Verification items for the finished model (mm, model axes). A direction names the side the tool comes from. Round coordinates to 2 decimals unless told otherwise and drop trailing zeros. Order: outer loops, then holes, each group sorted by start corner. A loop starts at its lowest first (then second) coordinate and runs counter-clockwise, first axis right, second up. Notation, with made-up numbers: M 17.5,43.5 L 35.5,43.5 A9 ccw 35.5,59.5 Z; hole C -2.5,2 d1. An arc over 180 degrees is marked long. Write item = value, one per line. Start each with the question number.
from build123d import *

# Parameters (mm, degrees)
F0_W      = 12.7
F0_H      = 12.7
F1_DEPTH  = 50.8
F3_DEPTH  = 25.4
F5_DEPTH  = 25.4
F7_DEPTH  = 12.7
F9_DEPTH  = 25.4
F12_DEPTH = 25.4
F13_W     = 40.64
F13_H     = 7.62
F15_W     = 7.62
F15_H     = 40.64
F11_W     = 7.62
F11_H     = 40.64
F14_W     = 40.64
F14_H     = 7.62
F16_DEPTH = 43.18


# Not quite as in the source:
# - a feature names something its author has since deleted; it is built from what else it names


with BuildPart() as f1:
    # F0 (on Top) → F1 (new body)
    with BuildSketch(Plane.XY):
        Polygon((0, 12.7), (0, 0), (31.75, 0), (38.0062268819, 0), (50.8, 0), (50.8, 12.7), (38.1, 12.7), (31.75, 12.7), align=None)
        Polygon((0, -5.08), (0, 0), (-12.7, 0), (-12.7, -5.08), (-12.7, -13.97), (-12.7, -16.51), (-12.7, -25.4), (-12.7, -31.75), (-12.7, -38.1), (-12.7, -50.8), (0, -50.8), (0, -38.0530845557), (0, -31.75), (0, -25.4), (0, -16.51), (0, -13.97), align=None)
        Polygon((-12.7, 12.7), (0, 12.7), (0, 17.78), (0, 26.67), (0, 29.21), (0, 38.1), (0, 44.45), (0, 50.8), (0, 63.5), (-12.7, 63.5), (-12.7, 50.8), (-12.7, 44.45), (-12.7, 38.1), (-12.7, 26.67), (-12.7, 17.78), align=None)
        Polygon((-44.45, 0), (-12.7, 0), (-12.7, 12.7), (-44.45, 12.7), (-50.8, 12.7), (-63.5, 12.7), (-63.5, 0), (-50.8, 0), align=None)
        with Locations((-6.35, 6.35)):
            Rectangle(F0_W, F0_H)
    extrude(amount=F1_DEPTH)

    # F2 (on face) → F3 (cut)
    with BuildSketch(Plane.XZ):
        Polygon((-63.5, 50.8), (-12.7, 25.4), (-12.7, 50.8), align=None)
    extrude(amount=-F3_DEPTH, mode=Mode.SUBTRACT)

    # F4 (on face) → F5 (cut)
    with BuildSketch(Plane(origin=(-12.7, 0, 0), x_dir=(0, -1, 0), z_dir=(-1, 0, 0))):
        Polygon((0, 50.8), (0, 25.4), (50.8, 50.8), align=None)
    extrude(amount=-F5_DEPTH, mode=Mode.SUBTRACT)

    # F6 (on face) → F7 (cut)
    with BuildSketch(Plane(origin=(-12.7, 0, 0), x_dir=(0, -1, 0), z_dir=(-1, 0, 0))):
        Polygon((-12.7, 25.4), (0, 25.4), (0, 50.8), (-63.5, 50.8), align=None)
    extrude(amount=-F7_DEPTH, mode=Mode.SUBTRACT)

    # F8 (on face) → F9 (cut)
    with BuildSketch(Plane(origin=(0, 12.7, 0), x_dir=(-1, 0, 0), z_dir=(0, 1, 0))):
        Polygon((-50.8, 50.8), (0, 25.4), (0, 50.8), align=None)
    extrude(amount=-F9_DEPTH, mode=Mode.SUBTRACT)

    # F0 (on Top) → F12 (join)
    with BuildSketch(Plane.XY):
        with BuildLine():
            Line((38.0062268819, 0), (31.75, 0))
            ThreePointArc((31.75, 0), (31.6475760941, -2.5482204312), (31.3409652053, -5.08))
            ThreePointArc((31.3409652053, -5.08), (30.2545088643, -9.6294960085), (28.5114292872, -13.97))
            ThreePointArc((28.5114292872, -13.97), (27.8445816489, -15.2558766643), (27.1197787602, -16.51))
            ThreePointArc((27.1197787602, -16.51), (23.5089375066, -21.339924023), (19.05, -25.4))
            ThreePointArc((19.05, -25.4), (10.040231571, -30.1206947131), (0, -31.75))
            Line((0, -31.75), (0, -38.0530845557))
            ThreePointArc((0, -38.0530845557), (26.8772997991, -26.8910325481), (38.0062268819, 0))
        make_face()
        with BuildLine():
            ThreePointArc((31.3409652053, 17.78), (31.6475760941, 15.2482204312), (31.75, 12.7))
            Line((31.75, 12.7), (38.1, 12.7))
            ThreePointArc((38.1, 12.7), (26.9407683632, 39.6407683632), (0, 50.8))
            Line((0, 50.8), (0, 44.45))
            ThreePointArc((0, 44.45), (10.040231571, 42.8206947131), (19.05, 38.1))
            ThreePointArc((19.05, 38.1), (23.5089375066, 34.039924023), (27.1197787602, 29.21))
            ThreePointArc((27.1197787602, 29.21), (27.8445816489, 27.9558766643), (28.5114292872, 26.67))
            ThreePointArc((28.5114292872, 26.67), (30.2545088643, 22.3294960085), (31.3409652053, 17.78))
        make_face()
        with BuildLine():
            Line((-12.7, -13.97), (-12.7, -5.08))
            Line((-12.7, -5.08), (-44.0409652053, -5.08))
            ThreePointArc((-44.0409652053, -5.08), (-44.3475760941, -2.5482204312), (-44.45, 0))
            Line((-44.45, 0), (-50.8, 0))
            ThreePointArc((-50.8, 0), (-39.6407683632, -26.9407683632), (-12.7, -38.1))
            Line((-12.7, -38.1), (-12.7, -31.75))
            ThreePointArc((-12.7, -31.75), (-22.740231571, -30.1206947131), (-31.75, -25.4))
            ThreePointArc((-31.75, -25.4), (-36.2089375066, -21.339924023), (-39.8197787602, -16.51))
            ThreePointArc((-39.8197787602, -16.51), (-40.5445816489, -15.2558766643), (-41.2114292872, -13.97))
            Line((-41.2114292872, -13.97), (-12.7, -13.97))
        make_face()
        with BuildLine():
            Line((-50.8, 12.7), (-44.45, 12.7))
            ThreePointArc((-44.45, 12.7), (-44.3475760941, 15.2482204312), (-44.0409652053, 17.78))
            ThreePointArc((-44.0409652053, 17.78), (-42.9545088643, 22.3294960085), (-41.2114292872, 26.67))
            ThreePointArc((-41.2114292872, 26.67), (-37.1577924997, 32.9454658143), (-31.75, 38.1))
            ThreePointArc((-31.75, 38.1), (-22.740231571, 42.8206947131), (-12.7, 44.45))
            Line((-12.7, 44.45), (-12.7, 50.8))
            ThreePointArc((-12.7, 50.8), (-39.6407683632, 39.6407683632), (-50.8, 12.7))
        make_face()
        with BuildLine():
            Line((-12.7, -25.4), (-12.7, -16.51))
            Line((-12.7, -16.51), (-39.8197787602, -16.51))
            ThreePointArc((-39.8197787602, -16.51), (-36.2089375066, -21.339924023), (-31.75, -25.4))
            Line((-31.75, -25.4), (-12.7, -25.4))
        make_face()
        with BuildLine():
            Line((0, 38.1), (0, 29.21))
            Line((0, 29.21), (27.1197787602, 29.21))
            ThreePointArc((27.1197787602, 29.21), (23.5089375066, 34.039924023), (19.05, 38.1))
            Line((19.05, 38.1), (0, 38.1))
        make_face()
        with BuildLine():
            Line((0, 26.67), (0, 17.78))
            Line((0, 17.78), (31.3409652053, 17.78))
            ThreePointArc((31.3409652053, 17.78), (30.2545088643, 22.3294960085), (28.5114292872, 26.67))
            Line((28.5114292872, 26.67), (0, 26.67))
        make_face()
        with BuildLine():
            Line((-41.2114292872, 26.67), (-12.7, 26.67))
            Line((-12.7, 26.67), (-12.7, 38.1))
            Line((-12.7, 38.1), (-31.75, 38.1))
            ThreePointArc((-31.75, 38.1), (-37.1577924997, 32.9454658143), (-41.2114292872, 26.67))
        make_face()
        with BuildLine():
            Line((-44.0409652053, 17.78), (-12.7, 17.78))
            Line((-12.7, 17.78), (-12.7, 26.67))
            Line((-12.7, 26.67), (-41.2114292872, 26.67))
            ThreePointArc((-41.2114292872, 26.67), (-42.9545088643, 22.3294960085), (-44.0409652053, 17.78))
        make_face()
        with BuildLine():
            Line((31.3409652053, -5.08), (0, -5.08))
            Line((0, -5.08), (0, -13.97))
            Line((0, -13.97), (28.5114292872, -13.97))
            ThreePointArc((28.5114292872, -13.97), (30.2545088643, -9.6294960085), (31.3409652053, -5.08))
        make_face()
        with BuildLine():
            Line((27.1197787602, -16.51), (0, -16.51))
            Line((0, -16.51), (0, -25.4))
            Line((0, -25.4), (19.05, -25.4))
            ThreePointArc((19.05, -25.4), (23.5089375066, -21.339924023), (27.1197787602, -16.51))
        make_face()
    extrude(amount=F12_DEPTH)

    # F13 (on offset) + F15 (on offset) + F11 (on offset) + F14 (on offset) → F16 (cut)
    with BuildSketch(Plane.XY.offset(52.324)):
        with Locations((22.1610166958, 6.35)):
            Rectangle(F13_W, F13_H)
    with BuildSketch(Plane.XY.offset(52.324)):
        with Locations((-6.35, -21.4313176799)):
            Rectangle(F15_W, F15_H)
    with BuildSketch(Plane.XY.offset(52.324)):
        with Locations((-6.35, 34.922975541)):
            Rectangle(F11_W, F11_H)
    with BuildSketch(Plane.XY.offset(52.324)):
        with Locations((-34.2408475804, 6.35)):
            Rectangle(F14_W, F14_H)
    extrude(amount=-F16_DEPTH, mode=Mode.SUBTRACT)


solid = f1.part
1) Scan lines: probe 1 along Y at (x, z) = (-8, 23.5); probe 2 along X at (y, z) = (4.5, 18); probe 3 along X at (y, z) = (-25, 26). Record each from-to range of solid material in increasing order.
2) Cross-section at C-C, the plane y = 5. Enter the section's corners in (x, z), then the cut area to 3 significant figures.
3) Cross-section at D-D, the plane x = -53. Enter the section's corners in (y, z), then the cut area to 3 significant figures.
4) Access from +Z, -Z, +X, -X, +Y, -Y to the whole of each face (thin tool, end or side, straight path). Record for faces 1 (the flat face through (19, -19, 25.4)), 2 (the flat face through (-12.7, -31, 25)), 3 (the flat face through (9, -25.4, 13)).
5) Cross-section at B-B, the plane x = 20.5. Enter the section's corners in (y, z), then the cut area to 3 significant figures.
6) Gauge pin test, flat ends, axial feed: P1, Ø10, axis at x = 8, z = 15, coming from the +Y side; P2, Ø3, axis at y = 51, z = 38.5, coming from the +X side; P3, Ø15, axis at y = 50.5, z = 24, coming from the +X side. Record the tip position at first contact, or that the pin passes through.
7) Release check for a two-part mould opening along Y. For faces 4 (the flat face through (-54.561, 6, 28)), 5 (the flat face through (-32, -19, 25.4)) record: pulls with the +Y half, pulls with the -Y half, needs draft (parallel to the pull), parting line crosses it, or undercut.
8) Cross-section at A-A, the plane z = 38.5. Give the number of separate pieces and of enclosed holes in the cut face, then the cut area to 3 significant figures.
Geometry results:
q1.probe_1 = -50.8 to -41.75, -1.11 to 14.6, 55.24 to 63.5
q1.probe_2 = -63.5 to -54.56, -13.92 to 1.84, 42.48 to 50.8
q1.probe_3 = -12.7 to -10.16, -2.54 to 0
q2.outline = M -63.5,0 L 50.8,0 L 50.8,50.8 L 42.48,46.64 L 42.48,9.14 L 1.84,9.14 L 1.84,26.32 L 0,25.4 L -12.7,25.4 L -13.92,26.01 L -13.92,9.14 L -54.56,9.14 L -54.56,46.33 L -63.5,50.8 Z
q2.area = 1,980 mm^2
q3.outline = M 0,0 L 12.7,0 L 12.7,45.55 L 10.16,45.55 L 10.16,9.14 L 2.54,9.14 L 2.54,45.55 L 0,45.55 Z
q3.area = 301 mm^2
q4.face_1 = +Z, +X, -Y
q4.face_2 = +Z
q4.face_3 = +Z, -Z
q5.outline = M -32.03,0 L -16.51,0 L -16.51,25.4 L -32.03,25.4 Z; M -13.97,0 L -5.08,0 L -5.08,25.4 L -13.97,25.4 Z; M 0,0 L 12.7,0 L 12.7,35.65 L 10.16,35.65 L 10.16,9.14 L 2.54,9.14 L 2.54,35.65 L 0,35.65 Z; M 17.78,0 L 26.67,0 L 26.67,25.4 L 17.78,25.4 Z; M 29.21,0 L 44.81,0 L 44.81,25.4 L 29.21,25.4 Z
q5.area = 1,490 mm^2
q6.P1 = 50.68
q6.P2 = 0
q6.P3 = 23.1
q7.face_4 = undercut
q7.face_5 = needs draft
q8.separate_pieces = 4
q8.enclosed_holes = 0
q8.area = 763 mm^2
